```python
from build123d import *

# Parameters (mm, degrees)
SKETCH_1_R          = 2
SKETCH_1_R_2        = 24.5
SKETCH_1_R_3        = 2.25
EXTRUDE_1_DEPTH     = 10
SKETCH_2_R          = 2
CUT_EXTRUDE_1_DEPTH = 15
SKETCH_4_R          = 4
CUT_EXTRUDE_3_DEPTH = 4


with BuildPart() as part:
    # 스케치1 → 보스-돌출1 (new body)
    with BuildSketch(Plane.XY):
        with BuildLine():
            Line((-39.5, 0), (-39.5, 42))
            Line((-39.5, 42), (39.5, 42))
            Line((39.5, 42), (39.5, 0))
            ThreePointArc((39.5, 0), (0, -39.5), (-39.5, 0))
        make_face()
        with Locations((0, -35.5)):
            Circle(SKETCH_1_R, mode=Mode.SUBTRACT)
        with Locations((-25.102290732, -25.102290732)):
            Circle(SKETCH_1_R, mode=Mode.SUBTRACT)
        with Locations((-35.5, 0)):
            Circle(SKETCH_1_R, mode=Mode.SUBTRACT)
        with Locations((-25.102290732, 25.102290732)):
            Circle(SKETCH_1_R, mode=Mode.SUBTRACT)
        with Locations((0, 35.5)):
            Circle(SKETCH_1_R, mode=Mode.SUBTRACT)
        with Locations((25.102290732, 25.102290732)):
            Circle(SKETCH_1_R, mode=Mode.SUBTRACT)
        with Locations((35.5, 0)):
            Circle(SKETCH_1_R, mode=Mode.SUBTRACT)
        with Locations((25.102290732, -25.102290732)):
            Circle(SKETCH_1_R, mode=Mode.SUBTRACT)
        Circle(SKETCH_1_R_2, mode=Mode.SUBTRACT)
        with Locations((-12.341540694, -29.795114923)):
            Circle(SKETCH_1_R_3, mode=Mode.SUBTRACT)
        with Locations((12.341540694, -29.795114923)):
            Circle(SKETCH_1_R_3, mode=Mode.SUBTRACT)
    extrude(amount=EXTRUDE_1_DEPTH)

    # 스케치2 → 컷-돌출1 (cut)
    with BuildSketch(Plane(origin=(0, 42, 0), x_dir=(1, 0, 0), z_dir=(0, 1, 0))):
        with Locations(Location((-30, -5, 0), (0, 0, 270))):
            Circle(SKETCH_2_R)
        with Locations(Location((-15, -5, 0), (0, 0, 270))):
            Circle(SKETCH_2_R)
        with Locations(Location((15, -5, 0), (0, 0, 270))):
            Circle(SKETCH_2_R)
        with Locations(Location((30, -5, 0), (0, 0, 270))):
            Circle(SKETCH_2_R)
    extrude(amount=-CUT_EXTRUDE_1_DEPTH, mode=Mode.SUBTRACT)

    # 스케치4 → 컷-돌출3 (cut)
    with BuildSketch(Plane.XY.offset(10)):
        with Locations((-12.341540694, -29.795114923)):
            Circle(SKETCH_4_R)
        with Locations((12.341540694, -29.795114923)):
            Circle(SKETCH_4_R)
    extrude(amount=-CUT_EXTRUDE_3_DEPTH, mode=Mode.SUBTRACT)


solid = part.part
```
For this review, take the finished solid that the model builds, in its own axes (mm). A direction names the side the tool comes from. Round coordinates to 2 decimals unless told otherwise and drop trailing zeros. Loops run counter-clockwise (first coordinate to the right, second up) from the corner with the lowest first, then second, coordinate; pieces in that order, holes last.
(1) We need section A-A (y = 35.5). Give the boundary of the cut face in (x, z).
Returned:
outline: (-39.5, 0) - (-2, 0) - (-2, 10) - (-39.5, 10) - close; (2, 0) - (39.5, 0) - (39.5, 10) - (2, 10) - close; hole circle Ø4 at (-30, 5); hole circle Ø4 at (-15, 5); hole circle Ø4 at (15, 5); hole circle Ø4 at (30, 5)
(2) We need section C-C (z = 5). State how many separate pieces and enclosed holes the cut face has, plus the area to 3 significant figures.
Returned:
separate pieces: 1
enclosed holes: 11
area: 3,510 mm2
(3) We need section D-D (y = 20.5). Give the boundary of the cut face in (x, z), plus the area to 3 significant figures.
Returned:
outline: (-39.5, 0) - (-13.42, 0) - (-13.42, 10) - (-39.5, 10) - close; (13.42, 0) - (39.5, 0) - (39.5, 10) - (13.42, 10) - close
area: 522 mm2
(4) Tool access review of faces 4 (the flat face through (-11, -32, 6)), 5 (the cylindrical face through (37.347, -0.766, 4.93)), 6 (the cylindrical face through (28, 35, 5)): name each direction out of +Z, -Z, +X, -X, +Y, -Y from which nothing blocks a thin tool from reaching the whole face with its end or side.
Returned:
face 4: +Z
face 5: +Z, -Z
face 6: +Y
(5) Clearance check with flat-ended pins moving along their axes: P1, Ø2, axis at x = 9, y = -20.5, coming from the +Z side; P2, Ø3.5, axis at x = 30, z = 5, coming from the +Y side; P3, Ø2.5, axis at x = 15, z = 5, coming from the -Y side; P4, Ø3, axis at y = -23.5, z = 3, coming from the -X side. State where each tip first meets the part, or that it passes through.
Returned:
P1: passes through
P2: stops at y = 27
P3: stops at y = -37.03
P4: stops at x = -32.81
(6) Wall thickness on line 1 along Y through (x, z) = (0, 4.25); line 2 along X through (y, z) = (35.75, 5); line 3 along X through (y, z) = (34, 5): over which ranges is each line inside the solid? List them lowest first.
Returned:
line 1: y = -39.5 to -37.5, -33.5 to -24.5, 24.5 to 33.5, 37.5 to 42
line 2: x = -39.5 to -32, -28 to -17, -13 to -1.98, 1.98 to 13, 17 to 28, 32 to 39.5
line 3: x = -39.5 to -32, -28 to -17, -13 to -1.32, 1.32 to 13, 17 to 28, 32 to 39.5
(7) Mouldability with a two-part tool opening along X and no side actions: class faces 1 (the flat face through (-1, 42, 5)), 2 (the flat face through (14, -32, 6)), 3 (the cylindrical face through (0.87, -39.49, 4.93)) as released by +X, released by -X, zero draft, split by the parting line, or undercut.
Returned:
face 1: zero draft
face 2: undercut
face 3: split by the parting line
(8) We need section B-B (x = 5.5). Give the boundary of the cut face in (y, z).
Returned:
outline: (-39.12, 0) - (-23.87, 0) - (-23.87, 10) - (-39.12, 10) - close; (23.87, 0) - (42, 0) - (42, 10) - (23.87, 10) - close
